from build123d import *

# Parameters (mm, degrees)
SKETCH_1_R      = 1.1
SKETCH_1_R_2    = 1.65
SKETCH_1_W      = 12.5
SKETCH_1_H      = 23
EXTRUDE_1_DEPTH = 3


with BuildPart() as part:
    # 草图1 → 凸台-拉伸1 (new body)
    with BuildSketch(Plane.XY):
        with BuildLine():
            Line((15, -25), (15, -5))
            Line((15, -5), (95, -5))
            ThreePointArc((95, -5), (100, 0), (95, 5))
            Line((95, 5), (15, 5))
            Line((15, 5), (15, 25))
            Line((15, 25), (-15, 25))
            Line((-15, 25), (-15, -25))
            Line((-15, -25), (15, -25))
        make_face()
        with Locations((0, 19.75)):
            Circle(SKETCH_1_R, mode=Mode.SUBTRACT)
        with Locations((0, -9.25)):
            Circle(SKETCH_1_R, mode=Mode.SUBTRACT)
        with Locations((95, 0)):
            Circle(SKETCH_1_R_2, mode=Mode.SUBTRACT)
        with Locations((10, 15)):
            Circle(SKETCH_1_R_2, mode=Mode.SUBTRACT)
        with Locations((-10, 15)):
            Circle(SKETCH_1_R_2, mode=Mode.SUBTRACT)
        with Locations(Location((10, -15, 0), (0, 0, 180))):
            Circle(SKETCH_1_R_2, mode=Mode.SUBTRACT)
        with Locations(Location((-10, -15, 0), (0, 0, 180))):
            Circle(SKETCH_1_R_2, mode=Mode.SUBTRACT)
        with Locations((0, 5.25)):
            Rectangle(SKETCH_1_W, SKETCH_1_H, mode=Mode.SUBTRACT)
        with BuildLine():
            Line((20, -1.65), (60, -1.65))
            ThreePointArc((60, -1.65), (61.65, 0), (60, 1.65))
            Line((60, 1.65), (20, 1.65))
            ThreePointArc((20, 1.65), (18.35, 0), (20, -1.65))
        make_face(mode=Mode.SUBTRACT)
    extrude(amount=EXTRUDE_1_DEPTH)


solid = part.part
Input: part model. Units: mm. Frame: model coordinates. A direction names the side the tool comes from. Give positions to 0.01 mm unless a question says otherwise; leave off trailing zeros. Write each loop counter-clockwise with the first axis right and the second up, starting at its lowest first coordinate (ties: lowest second). Pieces come first, ordered by that corner, then holes. Notation, with made-up numbers: M 73.5,60 L 123.5,60 A23 ccw 123.5,90 Z; hole C 70.25,63.5 d4. An arc over 180 degrees is marked long. Use one line per item in the form item = value.
1. Cut plane B-B on y = -15. Return loops of the section in (x, z), and give its area (3 significant figures).
Outcome:
outline = M -15,0 L -11.65,0 L -11.65,3 L -15,3 Z; M -8.35,0 L 8.35,0 L 8.35,3 L -8.35,3 Z; M 11.65,0 L 15,0 L 15,3 L 11.65,3 Z
area = 70.2 mm²
2. Cut plane C-C on y = 19.75. Return loops of the section in (x, z), and give its area (3 significant figures).
Outcome:
outline = M -15,0 L -1.1,0 L -1.1,3 L -15,3 Z; M 1.1,0 L 15,0 L 15,3 L 1.1,3 Z
area = 83.4 mm²
3. Mould query, pull axis Y, two halves, no side actions, for faces 6 (the face through (54, -5, 1)), 7 (the face through (40, 1.65, 1)), 8 (the face through (15, 15, 1)). Classes: released by +Y, released by -Y, zero draft, split by the parting line, or undercut.
Outcome:
face_6 = released by -Y
face_7 = undercut
face_8 = zero draft
4. Ray query, L1, parallel to Y at x = 0, z = 1.9; L2, parallel to Y at x = 10, z = 1.2; L3, parallel to X at y = -15, z = 0.95. Return the intervals inside material, ascending.
Outcome:
L1 = -25 to -10.35, -8.15 to -6.25, 16.75 to 18.65, 20.85 to 25
L2 = -25 to -16.65, -13.35 to 13.35, 16.65 to 25
L3 = -15 to -11.65, -8.35 to 8.35, 11.65 to 15
5. First-contact query: P1, Ø0.9, axis at y = 2.5, z = 1, coming from the +X side; P2, Ø1.5, axis at x = 68.5, z = 1.5, coming from the -Y side; P3, Ø0.9, axis at x = 34, z = 1, coming from the +Y side. Flat tips, straight axial feed; report the tip coordinate or a pass-through.
Outcome:
P1 = 99.56
P2 = -5
P3 = 5
6. Cut plane D-D on x = 37. Return loops of the section in (y, z).
Outcome:
outline = M -5,0 L -1.65,0 L -1.65,3 L -5,3 Z; M 1.65,0 L 5,0 L 5,3 L 1.65,3 Z
7. Reachability of faces 1 (the face through (56, 5, 1)), 2 (the face through (61.65, -0.04, 1.48)), 3 (the face through (15, -15, 1)), 4 (the face through (-15, 0, 1)), 5 (the face through (0, -25, 1)) from +Z, -Z, +X, -X, +Y, -Y: full face, straight path, thin tool, end or side. Return the list, or none.
Outcome:
face_1 = +Z, -Z, +X, +Y
face_2 = +Z, -Z
face_3 = +Z, -Z, +X, -Y
face_4 = +Z, -Z, -X, +Y, -Y
face_5 = +Z, -Z, +X, -X, -Y
8. Cut plane A-A on x = -10. Return loops of the section in (y, z).
Outcome:
outline = M -25,0 L -16.65,0 L -16.65,3 L -25,3 Z; M -13.35,0 L 13.35,0 L 13.35,3 L -13.35,3 Z; M 16.65,0 L 25,0 L 25,3 L 16.65,3 Z
